from build123d import *

# Parameters (mm, degrees)
F0_W     = 152.4
F0_H     = 82.55
F1_DEPTH = 19.05
F2_SIZE  = 6.35
F3_W     = 127
F3_H     = 57.15
F4_DEPTH = 25.4
F5_R     = 3.175
F6_DEPTH = 69.851
F7_R     = 3.175


with BuildPart() as f1:
    # F0 (on Top) → F1 (new body)
    with BuildSketch(Plane.XY):
        Rectangle(F0_W, F0_H)
    extrude(amount=F1_DEPTH)

    # F2
    f2_edges = [f1.edges().sort_by_distance(p)[0] for p in [
        (0, 41.275, 19.05),
        (-76.2, 0, 19.05),
        (0, -41.275, 19.05),
        (76.2, 0, 19.05),
    ]]
    chamfer(f2_edges, length=F2_SIZE)

    # F3 (on face) → F4 (join)
    with BuildSketch(Plane(origin=(0, 0, 0), x_dir=(1, 0, 0), z_dir=(0, 0, -1))):
        Rectangle(F3_W, F3_H)
    extrude(amount=F4_DEPTH)

    # F5 (on face) → F6 (cut, through all)
    with BuildSketch(Plane.XZ.offset(28.575)):
        with Locations((-50.8, -12.7)):
            Circle(F5_R)
        with Locations((0, -12.7)):
            Circle(F5_R)
        with Locations((50.8, -12.7)):
            Circle(F5_R)
    extrude(amount=-F6_DEPTH, mode=Mode.SUBTRACT)

    # F7
    f7_edges = [f1.edges().sort_by_distance(p)[0] for p in [
        (-63.5, -28.575, -12.7),
        (63.5, -28.575, -12.7),
        (-63.5, 28.575, -12.7),
        (63.5, 28.575, -12.7),
    ]]
    fillet(f7_edges, radius=F7_R)


solid = f1.part
For this review, take the finished solid that the model builds, in its own axes (mm). A direction names the side the tool comes from. Give positions to 0.01 mm unless a question says otherwise; leave off trailing zeros. Loops run counter-clockwise (first coordinate to the right, second up) from the corner with the lowest first, then second, coordinate; pieces in that order, holes last.
Item 1: Take a section at C-C, the plane x = 50.8. State the section outline as (y, z) points (3 decimals).
Item 2: Take a section at D-D, the plane x = 24. State the section outline as (y, z) points (3 decimals), and give its area (3 significant figures).
Item 3: Draft analysis for pull direction Z (two halves, no side actions). For faces 4 (the cylindrical face through (53.73, -0.4, -13.92)), 5 (the flat face through (-1, 28.575, -18)), 6 (the flat face through (-73, -0.6, 15.9)), state which applies: +Z half, -Z half, draft (parallel to the pull), parting line (faces both ways), or undercut.
Item 4: Take a section at B-B, the plane z = -12.7. State the section outline as (x, y) points (3 decimals).
Item 5: For line 1 along Z through (x, y) = (0, -0.5) (3 decimals); line 2 along X through (y, z) = (-2, -12); line 3 along Y through (x, z) = (59, -10.5) (3 decimals), list the stretches that pass through material, from the lowest coordinate up.
Item 6: Insertion check: pin 1 (8.5 mm diameter, centred on x = 50.8, z = -12.7, fed in from -Y) (3 decimals); pin 2 (7.5 mm diameter, centred on y = 2, z = -8.5, fed in from +X); pin 3 (8.5 mm diameter, centred on x = 0, z = -12.7, fed in from +Y) (3 decimals); pin 4 (4 mm diameter, centred on x = 16.5, y = 29, fed in from -Z). Each pin has a flat end and moves straight along its axis. Give the tip position at first contact, or say it passes through.
Item 7: Tool access review of faces 1 (the cylindrical face through (62.595, 27.62, -12.878)), 2 (the cylindrical face through (-62.595, -27.62, -12.878)), 3 (the flat face through (-63.5, 0, -13)): name each direction out of +Z, -Z, +X, -X, +Y, -Y from which nothing blocks a thin tool from reaching the whole face with its end or side.
Item 8: Take a section at A-A, the plane y = -16.5. State the section outline as (x, z) points (3 decimals), and give its area (3 significant figures).
Calculated:
1. outline: (-41.275, 0) - (-28.575, 0) - (-28.575, -9.525) - (28.575, -9.525) - (28.575, 0) - (41.275, 0) - (41.275, 12.7) - (34.925, 19.05) - (-34.925, 19.05) - (-41.275, 12.7) - close; (-28.575, -25.4) - (28.575, -25.4) - (28.575, -15.875) - (-28.575, -15.875) - close
2. outline: (-41.275, 0) - (-28.575, 0) - (-28.575, -25.4) - (28.575, -25.4) - (28.575, 0) - (41.275, 0) - (41.275, 12.7) - (34.925, 19.05) - (-34.925, 19.05) - (-41.275, 12.7) - close
2. area: 2,980 mm2
3. face 4: undercut
3. face 5: draft
3. face 6: +Z half
4. outline: (-63.5, -25.4) arc R3.175 ccw to (-60.325, -28.575) - (-53.975, -28.575) - (-53.975, 28.575) - (-60.325, 28.575) arc R3.175 ccw to (-63.5, 25.4) - close; (-47.625, -28.575) - (-3.175, -28.575) - (-3.175, 28.575) - (-47.625, 28.575) - close; (3.175, -28.575) - (47.625, -28.575) - (47.625, 28.575) - (3.175, 28.575) - close; (53.975, -28.575) - (60.325, -28.575) arc R3.175 ccw to (63.5, -25.4) - (63.5, 25.4) arc R3.175 ccw to (60.325, 28.575) - (53.975, 28.575) - close
5. line 1: z = -25.4 to -15.875, -9.525 to 19.05
5. line 2: x = -63.5 to -53.9, -47.7 to -3.1, 3.1 to 47.7, 53.9 to 63.5
5. line 3: y = -28.575 to 28.575
6. pin 1: stops at y = -28.575
6. pin 2: stops at x = 63.5
6. pin 3: stops at y = 28.575
6. pin 4: stops at z = -25.4
7. face 1: -Z, +X, +Y
7. face 2: -Z, -X, -Y
7. face 3: -Z, -X, +Y, -Y
8. outline: (-76.2, 0) - (-63.5, 0) - (-63.5, -25.4) - (63.5, -25.4) - (63.5, 0) - (76.2, 0) - (76.2, 12.7) - (69.85, 19.05) - (-69.85, 19.05) - (-76.2, 12.7) - close; hole circle Ø6.35 at (-50.8, -12.7); hole circle Ø6.35 at (0, -12.7); hole circle Ø6.35 at (50.8, -12.7)
8. area: 5,990 mm2
